Geometry: final body of the model. Coordinates: model frame, mm. Coordinates: 2 decimals unless noted, no trailing zeros. Write each loop counter-clockwise with the first axis right and the second up, starting at its lowest first coordinate (ties: lowest second). Pieces come first, ordered by that corner, then holes. Notation, with made-up numbers: (-33.5, 10.25) - (-8.5, 10.25) arc R34 ccw to (-8.5, 41.25) - close; hole circle Ø6 at (-3, 39). An arc over 180 degrees is marked (long way). Answer as a JSON object with one key per item and string values. Group by question number.
Item 1: Section A-A on y = -23. Return loops of the section in (x, z), and give its area (3 significant figures).
Item 2: Section C-C on x = -23. Return loops of the section in (y, z), and give its area (3 significant figures).
Item 3: Line query: line 1 along Y through (x, z) = (-23, 3.4); line 2 along Y through (x, z) = (24.5, 0.7); line 3 along Y through (x, z) = (5, 0.25). Output: solid intervals per line, ascending. Write a range as from..to.
Item 4: First-contact query: pin 1 Ø4 at (x, y) = (-23, 23) entering from +Z. Flat tip, straight axial feed; report the tip coordinate or a pass-through.
Item 5: Mould query, pull axis X, two halves, no side actions, for faces 1 (the flat face through (9, 29, 2)), 2 (the cylindrical face through (8.767, -16.856, 2.535)), 3 (the flat face through (-29, 0, 2)). Classes: pulls with the +X half, pulls with the -X half, needs draft (parallel to the pull), parting line crosses it, or undercut.
Item 6: Section B-B on z = 4. Return loops of the section in (x, y), and give its area (3 significant figures).
Item 7: Section D-D on y = -4.5. Return loops of the section in (x, z).
```python
from build123d import *

# Parameters (mm, degrees)
EXTRUDE_1_DEPTH     = 5
HOLE_WIZARD_M4_1_D  = 3.3
SKETCH_5_R          = 19
CUT_EXTRUDE_1_DEPTH = 54.768020235


with BuildPart() as part:
    # 草图1 → 凸台-拉伸1 (new body)
    with BuildSketch(Plane.XY):
        Polygon((29, 29), (45, 29), (45, -29), (29, -29), (-29, -29), (-29, 29), align=None)
    extrude(amount=EXTRUDE_1_DEPTH)

    # M4 螺纹孔的螺纹孔钻头1 (through all)
    with Locations(Plane(origin=(-23, 23, 5), x_dir=(1, 0, 0), z_dir=(0, 0, 1))):
        with Locations((0, 0), (46, 0)):
            hole_wizard_m4_1 = Hole(HOLE_WIZARD_M4_1_D / 2)

    # 镜向1: M4 螺纹孔的螺纹孔钻头1 across plane
    add(hole_wizard_m4_1.mirror(Plane.ZX), mode=Mode.SUBTRACT)

    # 草图5 → 切除-拉伸1 (cut, through all)
    with BuildSketch(Plane.XY.offset(5)):
        Circle(SKETCH_5_R)
    extrude(amount=-CUT_EXTRUDE_1_DEPTH, mode=Mode.SUBTRACT)


solid = part.part
```
Checks:
{
 "1": {"outline": "(-29, 0) - (-24.65, 0) - (-24.65, 5) - (-29, 5) - close; (-21.35, 0) - (21.35, 0) - (21.35, 5) - (-21.35, 5) - close; (24.65, 0) - (45, 0) - (45, 5) - (24.65, 5) - close", "area": "337 mm^2"},
 "2": {"outline": "(-29, 0) - (-24.65, 0) - (-24.65, 5) - (-29, 5) - close; (-21.35, 0) - (21.35, 0) - (21.35, 5) - (-21.35, 5) - close; (24.65, 0) - (29, 0) - (29, 5) - (24.65, 5) - close", "area": "257 mm^2"},
 "3": {"line 1": "-29..-24.65, -21.35..21.35, 24.65..29", "line 2": "-29..-23.69, -22.31..22.31, 23.69..29", "line 3": "-29..-18.33, 18.33..29"},
 "4": {"pin 1": "z = 5"},
 "5": {"face 1": "needs draft", "face 2": "undercut", "face 3": "pulls with the -X half"},
 "6": {"outline": "(-29, -29) - (45, -29) - (45, 29) - (-29, 29) - close; hole circle Ø3.3 at (-23, -23); hole circle Ø3.3 at (-23, 23); hole circle Ø38 at (0, 0); hole circle Ø3.3 at (23, -23); hole circle Ø3.3 at (23, 23)", "area": "3,120 mm^2"},
 "7": {"outline": "(-29, 0) - (-18.46, 0) - (-18.46, 5) - (-29, 5) - close; (18.46, 0) - (45, 0) - (45, 5) - (18.46, 5) - close"}
}
